```python
from build123d import *

# Parameters (mm, degrees)
BOSS_EXTRUDE1_DEPTH = 2.5


with BuildPart() as part:
    # Sketch1 → Boss-Extrude1 (new, symmetric)
    with BuildSketch(Plane(origin=(0, 0, 0), x_dir=(1, 0, 0), z_dir=(0, 1, 0))):
        Polygon((55, 45), (45, 45), (45, 40), (35, 40), (35, 45), (25, 45), (25, 40), (15, 40), (15, 45), (5, 45), (5, 40), (-5, 40), (-5, 45), (-15, 45), (-15, 40), (-25, 40), (-25, 45), (-35, 45), (-35, 40), (-45, 40), (-45, 45), (-55, 45), (-55, 40), (-55, 35), (-60, 35), (-60, 25), (-55, 25), (-55, 15), (-60, 15), (-60, 5), (-55, 5), (-55, -5), (-60, -5), (-60, -15), (-55, -15), (-55, -25), (-60, -25), (-60, -35), (-55, -35), (-55, -40), (-55, -45), (-45, -45), (-45, -40), (-35, -40), (-35, -45), (-25, -45), (-25, -40), (-15, -40), (-15, -45), (-5, -45), (-5, -40), (5, -40), (5, -45), (15, -45), (15, -40), (25, -40), (25, -45), (35, -45), (35, -40), (45, -40), (45, -45), (55, -45), (55, -40), (55, -35), (60, -35), (60, -25), (55, -25), (55, -15), (60, -15), (60, -5), (55, -5), (55, 5), (60, 5), (60, 15), (55, 15), (55, 25), (60, 25), (60, 35), (55, 35), (55, 40), align=None)
    extrude(amount=BOSS_EXTRUDE1_DEPTH, both=True)


solid = part.part
```
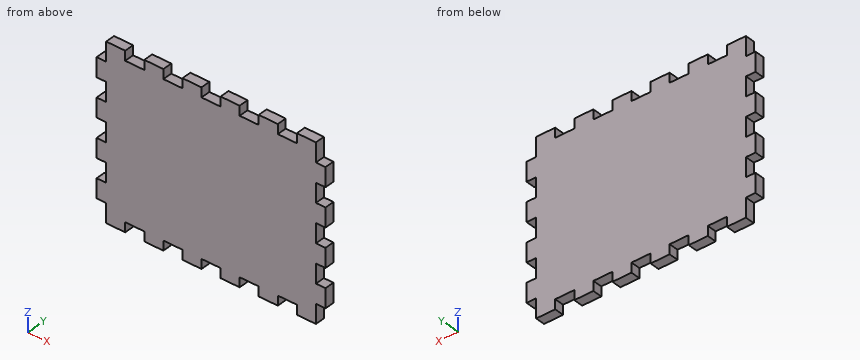
Geometry: final body of the model. Coordinates: model frame, mm. Round coordinates to 2 decimals unless told otherwise and drop trailing zeros. Write each loop counter-clockwise with the first axis right and the second up, starting at its lowest first coordinate (ties: lowest second). Pieces come first, ordered by that corner, then holes.
Item 1: Section query A-A (x = -17.5). Return loops of the section in (y, z), plus the area to 3 significant figures.
Item 2: Section query B-B (z = 1.5). Return loops of the section in (x, y), plus the area to 3 significant figures.
Item 3: Material intervals for L1, parallel to Z at x = -22.5, y = -1.5; L2, parallel to X at y = 0.5, z = -20, sorted ascending.
Item 4: Pin query (flat end, axial travel): P1, Ø1.5, axis at y = -1, z = -41.5, coming from the -X side; P2, Ø1.5, axis at y = 0.5, z = -42, coming from the +X side; P3, Ø1.5, axis at x = -57.5, y = -1, coming from the -Z side. Return the tip coordinate at first contact, or that it passes through.
Completed:
1. outline: (-2.5, -40) - (2.5, -40) - (2.5, 40) - (-2.5, 40) - close
1. area: 400 mm2
2. outline: (-55, -2.5) - (55, -2.5) - (55, 2.5) - (-55, 2.5) - close
2. area: 550 mm2
3. L1: z = -40 to 40
3. L2: x = -55 to 55
4. P1: stops at x = -55
4. P2: stops at x = 55
4. P3: stops at z = -35
